Read the model definition and answer for the solid it produces. Units are mm, in the model's axes. A direction names the side the tool comes from. Coordinates: 2 decimals unless noted, no trailing zeros. Write each loop counter-clockwise with the first axis right and the second up, starting at its lowest first coordinate (ties: lowest second). Pieces come first, ordered by that corner, then holes. Notation, with made-up numbers: (20.25, 78.5) - (77.25, 78.5) arc R22 cw to (77.25, 116.5) - close; hole circle Ø8 at (-13.75, 36.25). An arc over 180 degrees is marked (long way). Return JSON: item names as keys, results as strings.
```python
from build123d import *

# Parameters (mm, degrees)
SKETCH_1_W          = 9.5
SKETCH_1_H          = 6.52
EXTRUDE_1_DEPTH     = 2
SKETCH_2_W          = 14.5
SKETCH_2_H          = 16.02
EXTRUDE_2_DEPTH     = 1.5
SKETCH_3_R          = 1.1
CUT_EXTRUDE_1_DEPTH = 14.864587318
FILLET_3_R          = 0.8
FILLET_4_R          = 0.5
FILLET_7_R          = 0.15
FILLET_8_R          = 0.8
FILLET_10_R         = 0.3
SKETCH_4_R          = 2.1
CUT_EXTRUDE_2_DEPTH = 14.563804108
FILLET_11_R         = 0.3
FILLET_12_R         = 0.15


with BuildPart() as part:
    # Эскиз1 → Бобышка-Вытянуть1 (new body)
    with BuildSketch(Plane(origin=(0, 0, 0), x_dir=(1, 0, 0), z_dir=(0, 1, 0))):
        with Locations((1.785821709, 2.843815878)):
            Rectangle(SKETCH_1_W, SKETCH_1_H)
    extrude(amount=EXTRUDE_1_DEPTH)

    # Эскиз2 → Бобышка-Вытянуть2 (add)
    with BuildSketch(Plane(origin=(0, 2, 0), x_dir=(1, 0, 0), z_dir=(0, 1, 0))):
        with Locations((1.785821709, -1.906184122)):
            Rectangle(SKETCH_2_W, SKETCH_2_H)
    extrude(amount=EXTRUDE_2_DEPTH)

    # Эскиз3 → Вырез-Вытянуть1 (cut, through all)
    with BuildSketch(Plane(origin=(0, 3.5, 0), x_dir=(1, 0, 0), z_dir=(0, 1, 0))):
        with Locations(Location((1.785821709, -0.196184122, 0), (0, 0, 270))):
            Circle(SKETCH_3_R)
    extrude(amount=-CUT_EXTRUDE_1_DEPTH, mode=Mode.SUBTRACT)

    # Скругление3
    fillet_3_edges = [part.edges().sort_by_distance(p)[0] for p in [
        (-5.464178291, 3.5, 1.906184122),
        (1.785821709, 3.5, 9.916184122),
        (9.035821709, 3.5, 1.906184122),
        (1.785821709, 3.5, -6.103815878),
    ]]
    fillet(fillet_3_edges, radius=FILLET_3_R)

    # Скругление4
    fillet_4_edges = [part.edges().sort_by_distance(p)[0] for p in [
        (-2.964178291, 1, -6.103815878),
        (6.535821709, 1, -6.103815878),
        (6.535821709, 1, 0.416184122),
        (-2.964178291, 1, 0.416184122),
    ]]
    fillet(fillet_4_edges, radius=FILLET_4_R)

    # Скругление7
    fillet_7_edges = [part.edges().sort_by_distance(p)[0] for p in [
        (-5.464178291, 2, 1.906184122),
        (1.785821709, 2, 9.916184122),
        (9.035821709, 2, 1.906184122),
        (7.535821709, 2, -6.103815878),
        (-3.964178291, 2, -6.103815878),
    ]]
    fillet(fillet_7_edges, radius=FILLET_7_R)

    # Скругление8
    # the kernel refuses this fillet: 0.8 mm, written as the material it takes off along each edge
    with BuildSketch(Plane(origin=(-4.664178291, 2, -5.303815878), x_dir=(-1, 0, 0), z_dir=(0, 0, 1))) as fillet_8_piece_1:
        with BuildLine():
            CenterArc((0.65, -0.15), 0.15, 0, 90)
            Line((0.8, -0.15), (0.8, 0))
            Line((0.8, 0), (0.65, 0))
        make_face()
    revolve(axis=Axis((-4.664178291, 2, -5.303815878), (0, -1, 0)), revolution_arc=90, mode=Mode.SUBTRACT)
    with BuildSketch(Plane(origin=(-4.664178291, 2, 9.116184122), x_dir=(0, 0, 1), z_dir=(1, 0, 0))) as fillet_8_piece_2:
        with BuildLine():
            CenterArc((0.65, -0.15), 0.15, 0, 90)
            Line((0.8, -0.15), (0.8, 0))
            Line((0.8, 0), (0.65, 0))
        make_face()
    revolve(axis=Axis((-4.664178291, 2, 9.116184122), (0, -1, 0)), revolution_arc=90, mode=Mode.SUBTRACT)
    with BuildSketch(Plane(origin=(8.235821709, 2, 9.116184122), x_dir=(1, 0, 0), z_dir=(0, 0, -1))) as fillet_8_piece_3:
        with BuildLine():
            CenterArc((0.65, -0.15), 0.15, 0, 90)
            Line((0.8, -0.15), (0.8, 0))
            Line((0.8, 0), (0.65, 0))
        make_face()
    revolve(axis=Axis((8.235821709, 2, 9.116184122), (0, -1, 0)), revolution_arc=90, mode=Mode.SUBTRACT)
    with BuildSketch(Plane(origin=(8.235821709, 2, -5.303815878), x_dir=(0, 0, -1), z_dir=(-1, 0, 0))) as fillet_8_piece_4:
        with BuildLine():
            CenterArc((0.65, -0.15), 0.15, 0, 90)
            Line((0.8, -0.15), (0.8, 0))
            Line((0.8, 0), (0.65, 0))
        make_face()
    revolve(axis=Axis((8.235821709, 2, -5.303815878), (0, -1, 0)), revolution_arc=90, mode=Mode.SUBTRACT)
    with BuildSketch(Plane(origin=(8.235821709, 2.7, 9.116184122), x_dir=(1, 0, 0), z_dir=(0, 0, 1))) as fillet_8_piece_5_section:
        Polygon((0, 0), (FILLET_8_R, 0), (FILLET_8_R, FILLET_8_R), (0, FILLET_8_R), align=None)
    fillet_8_piece_5 = extrude(amount=FILLET_8_R, mode=Mode.PRIVATE)
    fillet_8_piece_5 = fillet_8_piece_5 - Plane(origin=(8.235821709, 2.7, 9.116184122), x_dir=(-0.7071067811865475, -0.7071067811865475, 0), z_dir=(0, 0, 1)) * Sphere(FILLET_8_R, mode=Mode.PRIVATE)
    add(fillet_8_piece_5, mode=Mode.SUBTRACT)
    with BuildSketch(Plane(origin=(-4.664178291, 2.7, 9.116184122), x_dir=(-1, 0, 0), z_dir=(0, 0, 1))) as fillet_8_piece_6_section:
        Polygon((0, 0), (FILLET_8_R, 0), (FILLET_8_R, -FILLET_8_R), (0, -FILLET_8_R), align=None)
    fillet_8_piece_6 = extrude(amount=FILLET_8_R, mode=Mode.PRIVATE)
    fillet_8_piece_6 = fillet_8_piece_6 - Plane(origin=(-4.664178291, 2.7, 9.116184122), x_dir=(0.7071067811865475, -0.7071067811865475, 0), z_dir=(0, 0, 1)) * Sphere(FILLET_8_R, mode=Mode.PRIVATE)
    add(fillet_8_piece_6, mode=Mode.SUBTRACT)
    with BuildSketch(Plane(origin=(8.235821709, 2.7, -5.303815878), x_dir=(1, 0, 0), z_dir=(0, 0, -1))) as fillet_8_piece_7_section:
        Polygon((0, 0), (FILLET_8_R, 0), (FILLET_8_R, -FILLET_8_R), (0, -FILLET_8_R), align=None)
    fillet_8_piece_7 = extrude(amount=FILLET_8_R, mode=Mode.PRIVATE)
    fillet_8_piece_7 = fillet_8_piece_7 - Plane(origin=(8.235821709, 2.7, -5.303815878), x_dir=(-0.7071067811865475, -0.7071067811865475, 0), z_dir=(0, 0, -1)) * Sphere(FILLET_8_R, mode=Mode.PRIVATE)
    add(fillet_8_piece_7, mode=Mode.SUBTRACT)
    with BuildSketch(Plane(origin=(-4.664178291, 2.7, -5.303815878), x_dir=(-1, 0, 0), z_dir=(0, 0, -1))) as fillet_8_piece_8_section:
        Polygon((0, 0), (FILLET_8_R, 0), (FILLET_8_R, FILLET_8_R), (0, FILLET_8_R), align=None)
    fillet_8_piece_8 = extrude(amount=FILLET_8_R, mode=Mode.PRIVATE)
    fillet_8_piece_8 = fillet_8_piece_8 - Plane(origin=(-4.664178291, 2.7, -5.303815878), x_dir=(0.7071067811865475, -0.7071067811865475, 0), z_dir=(0, 0, -1)) * Sphere(FILLET_8_R, mode=Mode.PRIVATE)
    add(fillet_8_piece_8, mode=Mode.SUBTRACT)
    with BuildSketch(Plane(origin=(-5.464178291, 2, -6.103815878), x_dir=(1, 0, 0), z_dir=(0, 1, 0)), Plane(origin=(9.035821709, 2, 9.916184122), x_dir=(-1, 0, 0), z_dir=(0, 1, 0))) as fillet_8_piece_9:
        with BuildLine():
            CenterArc((FILLET_8_R, -FILLET_8_R), FILLET_8_R, 90, 90)
            Line((0, -FILLET_8_R), (0, 0))
            Line((0, 0), (FILLET_8_R, 0))
        make_face()
    extrude(amount=0.7, mode=Mode.SUBTRACT)
    with BuildSketch(Plane(origin=(9.035821709, 2, -6.103815878), x_dir=(-1, 0, 0), z_dir=(0, 1, 0)), Plane(origin=(-5.464178291, 2, 9.916184122), x_dir=(1, 0, 0), z_dir=(0, 1, 0))) as fillet_8_piece_10:
        with BuildLine():
            CenterArc((FILLET_8_R, FILLET_8_R), FILLET_8_R, 180, 90)
            Line((0, FILLET_8_R), (0, 0))
            Line((0, 0), (FILLET_8_R, 0))
        make_face()
    extrude(amount=0.7, mode=Mode.SUBTRACT)

    # Скругление10
    fillet_10_edges = [part.edges().sort_by_distance(p)[0] for p in [
        (1.785821709, 3.5, -0.903815878),
    ]]
    fillet(fillet_10_edges, radius=FILLET_10_R)

    # Эскиз4 → Вырез-Вытянуть2 (cut, through all)
    with BuildSketch(Plane.XZ.offset(-2)):
        with Locations((1.785821709, 0.196184122)):
            Circle(SKETCH_4_R)
    extrude(amount=CUT_EXTRUDE_2_DEPTH, mode=Mode.SUBTRACT)

    # Скругление11
    fillet_11_edges = [part.edges().sort_by_distance(p)[0] for p in [
        (1.785821709, 0, -1.903815878),
        (-0.302622688, 1, 0.416184122),
        (3.874266106, 1, 0.416184122),
    ]]
    fillet(fillet_11_edges, radius=FILLET_11_R)

    # Скругление12
    fillet_12_edges = [part.edges().sort_by_distance(p)[0] for p in [
        (5.110154857, 0, 0.416184122),
        (-0.608464555, 0, 0.416152145),
        (4.180107973, 0, 0.416152145),
        (-0.383168508, 0.105102909, 0.309183864),
        (3.954811922, 0.10510291, 0.309183857),
        (-1.538511439, 0, 0.416184122),
        (-2.964178291, 0, -2.843815878),
        (1.785821709, 0, -6.103815878),
        (6.535821709, 0, -2.843815878),
        (-2.817731681, 0, -5.957369269),
        (6.3893751, 0, -5.957369269),
        (6.3893751, 0, 0.269737512),
        (-2.817731681, 0, 0.269737512),
    ]]
    fillet(fillet_12_edges, radius=FILLET_12_R)


solid = part.part
```
(1) A cutting plane is placed at A-A (x = 7). Determine the outline of the cut face in (y, z), and give its area (3 significant figures).
Answer:
{"outline": "(2, -5.95) arc R0.15 ccw to (2.15, -6.1) - (2.7, -6.1) arc R0.8 ccw to (3.5, -5.3) - (3.5, 9.12) arc R0.8 ccw to (2.7, 9.92) - (2.15, 9.92) arc R0.15 ccw to (2, 9.77) - close", "area": "23.7 mm²"}
(2) A cutting plane is placed at D-D (y = 3). Determine the outline of the cut face in (x, z).
Answer:
{"outline": "(-5.41, -5.3) arc R0.74 ccw to (-4.66, -6.05) - (8.24, -6.05) arc R0.74 ccw to (8.98, -5.3) - (8.98, 9.12) arc R0.74 ccw to (8.24, 9.86) - (-4.66, 9.86) arc R0.74 ccw to (-5.41, 9.12) - close; hole circle Ø2.2 at (1.79, 0.2)"}
(3) A cutting plane is placed at B-B (z = -4). Determine the outline of the cut face in (x, y).
Answer:
{"outline": "(-5.46, 2.15) arc R0.15 ccw to (-5.31, 2) - (-2.96, 2) - (-2.96, 0.15) arc R0.15 ccw to (-2.81, 0) - (6.39, 0) arc R0.15 ccw to (6.54, 0.15) - (6.54, 2) - (8.89, 2) arc R0.15 ccw to (9.04, 2.15) - (9.04, 2.7) arc R0.8 ccw to (8.24, 3.5) - (-4.66, 3.5) arc R0.8 ccw to (-5.46, 2.7) - close"}
(4) Straight lines are drawn through the part: line 1 (Y direction, x = -1.5, z = 7.25); line 2 (X direction, y = 1.3, z = -5.25); line 3 (X direction, y = 1.8, z = -1.25). For each, find the intervals that lie inside material, in ascending order. Write a range as from..to.
Answer:
{"line 1": "2..3.5", "line 2": "-2.96..6.54", "line 3": "-2.96..0.26, 3.31..6.54"}
(5) Flat-ended cylindrical pins translate along their axes: P1, Ø0.9, axis at x = -1.5, y = 1, coming from the +Z side; P2, Ø1.3, axis at x = 1.79, z = 0.2, coming from the -Y side; P3, Ø3, axis at x = 2, z = 4, coming from the -Y side; P4, Ø0.9, axis at y = 1, z = -3, coming from the -X side. Find the tip coordinate at first contact, or state that the pin passes through.
Answer:
{"P1": "z = 0.42", "P2": "through", "P3": "y = 2", "P4": "x = -2.96"}
(6) Determine the mould class of faces 4 (the face through (8.8, 3.27, 1.81)), 5 (the face through (2, 1, -6.104)), 6 (the face through (-5.236, 2.421, 9.676)), 7 (the face through (1.741, 1.162, -1.903)) for opening direction X: +X half, -X half, draft (parallel to the pull), parting line (faces both ways), or undercut.
Answer:
{"face 4": "+X half", "face 5": "draft", "face 6": "-X half", "face 7": "undercut"}
(7) Which of the six approach directions +Z, -Z, +X, -X, +Y, -Y give full straight-line access (tool end or side, diameter ignored) to faces 1 (the face through (-2.964, 1, -3)), 2 (the face through (-2, 1, 0.416)), 3 (the face through (6.536, 1, -3))?
Answer:
{"face 1": "+Z, -Z, -X, -Y", "face 2": "+Z, +X, -X, -Y", "face 3": "+Z, -Z, +X, -Y"}
(8) A cutting plane is placed at C-C (y = 1.75). Determine the outline of the cut face in (x, z), and give its area (3 significant figures).
Answer:
{"outline": "(-2.96, -5.6) arc R0.5 ccw to (-2.46, -6.1) - (6.04, -6.1) arc R0.5 ccw to (6.54, -5.6) - (6.54, -0.08) arc R0.5 ccw to (6.04, 0.42) - (4.18, 0.42) arc R0.3 ccw to (3.88, 0.13) arc R2.1 cw to (-0.31, 0.13) arc R0.3 ccw to (-0.61, 0.42) - (-2.46, 0.42) arc R0.5 ccw to (-2.96, -0.08) - close", "area": "53.8 mm²"}
